from build123d import *

# Parameters (mm, degrees)
SALIENTE_EXTRUIR1_DEPTH = 107
CORTAR_EXTRUIR1_REACH   = 40
CROQUIS3_R              = 2.5
CORTAR_EXTRUIR2_REACH   = 40
CROQUIS4_R              = 2.5


with BuildPart() as part:
    # Croquis1 → Saliente-Extruir1 (new body)
    with BuildSketch(Plane.XY):
        Polygon((0, 0), (9, 0), (17.5, 10.5), (17.5, 24.5), (9, 35), (0, 35), (0, 36.5), (9.715608012, 36.5), (19, 25.031045192), (19, 9.968954808), (9.715608012, -1.5), (0, -1.5), align=None)
    extrude(amount=SALIENTE_EXTRUIR1_DEPTH)

    # Croquis3 → Cortar-Extruir1 (cut, up to next)
    with BuildSketch(Plane(origin=(0, 36.5, 0), x_dir=(1, 0, 0), z_dir=(0, 1, 0)), mode=Mode.PRIVATE) as cortar_extruir1_sk1:
        with Locations((5, -8)):
            Circle(CROQUIS3_R)
    cortar_extruir1_tool1 = extrude(cortar_extruir1_sk1.sketch, amount=-CORTAR_EXTRUIR1_REACH, mode=Mode.PRIVATE) & part.part
    add(cortar_extruir1_tool1.solids().sort_by_distance((5, 36.5, 8))[0], mode=Mode.SUBTRACT)
    # Croquis3 → Cortar-Extruir1 (cut, up to next)
    with BuildSketch(Plane(origin=(0, 36.5, 0), x_dir=(1, 0, 0), z_dir=(0, 1, 0)), mode=Mode.PRIVATE) as cortar_extruir1_sk2:
        with Locations((5, -99)):
            Circle(CROQUIS3_R)
    cortar_extruir1_tool2 = extrude(cortar_extruir1_sk2.sketch, amount=-CORTAR_EXTRUIR1_REACH, mode=Mode.PRIVATE) & part.part
    add(cortar_extruir1_tool2.solids().sort_by_distance((5, 36.5, 99))[0], mode=Mode.SUBTRACT)

    # Croquis4 → Cortar-Extruir2 (cut, up to next)
    with BuildSketch(Plane.XZ.offset(1.5), mode=Mode.PRIVATE) as cortar_extruir2_sk1:
        with Locations((5, 8)):
            Circle(CROQUIS4_R)
    cortar_extruir2_tool1 = extrude(cortar_extruir2_sk1.sketch, amount=-CORTAR_EXTRUIR2_REACH, mode=Mode.PRIVATE) & part.part
    add(cortar_extruir2_tool1.solids().sort_by_distance((5, -1.5, 8))[0], mode=Mode.SUBTRACT)
    # Croquis4 → Cortar-Extruir2 (cut, up to next)
    with BuildSketch(Plane.XZ.offset(1.5), mode=Mode.PRIVATE) as cortar_extruir2_sk2:
        with Locations((5, 99)):
            Circle(CROQUIS4_R)
    cortar_extruir2_tool2 = extrude(cortar_extruir2_sk2.sketch, amount=-CORTAR_EXTRUIR2_REACH, mode=Mode.PRIVATE) & part.part
    add(cortar_extruir2_tool2.solids().sort_by_distance((5, -1.5, 99))[0], mode=Mode.SUBTRACT)


solid = part.part
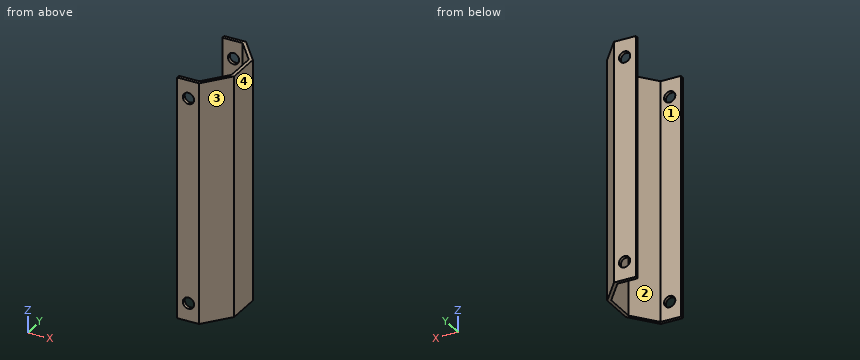
For this review, take the finished solid that the model builds, in its own axes (mm). Face numbers are marked on the shaded views. Round coordinates to 2 decimals unless told otherwise and drop trailing zeros. Loops run counter-clockwise (first coordinate to the right, second up) from the corner with the lowest first, then second, coordinate; pieces in that order, holes last. Notation, with made-up numbers: (21, -13) - (76, -13) arc R11 cw to (76, -3) - close; hole circle Ø2 at (-28.75, 29). An arc over 180 degrees is marked (long way). Put each result on its own line as item: value. Start each with the question number.
1. For probe 1 along Z at (x, y) = (5, 35.6); probe 2 along Y at (x, z) = (3, 96.5); probe 3 along X at (y, z) = (35.95, 8), list the stretches that pass through material, from the lowest coordinate up. Write a range as [from, to].
2. Consider section C-C on z = 58.5. State the section outline as (x, y) points, plus the area to 3 significant figures.
3. Consider section A-A on x = 5. State the section outline as (y, z) points, plus the area to 3 significant figures.
4. Consider section D-D on x = 15. State the section outline as (y, z) points, plus the area to 3 significant figures.
5. Insertion check: P1, Ø1, axis at y = 25, z = 40, coming from the -X side; P2, Ø4, axis at y = 15, z = 76.5, coming from the -X side. Each pin has a flat end and moves straight along its axis. Give the tip position at first contact, or say it passes through.
6. Consider section B-B on z = 99. State the section outline as (x, y) points, plus the area to 3 significant figures.
7. Mouldability with a two-part tool opening along Y and no side actions: class the marked faces 1, 2, 3 and 4 as +Y half, -Y half, draft (parallel to the pull), parting line (faces both ways), or undercut.
Result sheet:
1. probe 1: [0, 5.5], [10.5, 96.5], [101.5, 107]
1. probe 2: [-1.5, 0], [35, 36.5]
1. probe 3: [0, 2.5], [7.5, 10.16]
2. outline: (0, -1.5) - (9.72, -1.5) - (19, 9.97) - (19, 25.03) - (9.72, 36.5) - (0, 36.5) - (0, 35) - (9, 35) - (17.5, 24.5) - (17.5, 10.5) - (9, 0) - (0, 0) - close
2. area: 92.3 mm^2
3. outline: (-1.5, 0) - (0, 0) - (0, 5.5) - (-1.5, 5.5) - close; (-1.5, 10.5) - (0, 10.5) - (0, 96.5) - (-1.5, 96.5) - close; (-1.5, 101.5) - (0, 101.5) - (0, 107) - (-1.5, 107) - close; (35, 0) - (36.5, 0) - (36.5, 5.5) - (35, 5.5) - close; (35, 10.5) - (36.5, 10.5) - (36.5, 96.5) - (35, 96.5) - close; (35, 101.5) - (36.5, 101.5) - (36.5, 107) - (35, 107) - close
3. area: 291 mm^2
4. outline: (5.03, 0) - (7.41, 0) - (7.41, 107) - (5.03, 107) - close; (27.59, 0) - (29.97, 0) - (29.97, 107) - (27.59, 107) - close
4. area: 510 mm^2
5. P1: x = 16.69
5. P2: x = 17.5
6. outline: (0, -1.5) - (2.5, -1.5) - (2.5, 0) - (0, 0) - close; (0, 35) - (2.5, 35) - (2.5, 36.5) - (0, 36.5) - close; (7.5, -1.5) - (9.72, -1.5) - (19, 9.97) - (19, 25.03) - (9.72, 36.5) - (7.5, 36.5) - (7.5, 35) - (9, 35) - (17.5, 24.5) - (17.5, 10.5) - (9, 0) - (7.5, 0) - close
6. area: 77.3 mm^2
7. face 1: undercut
7. face 2: undercut
7. face 3: -Y half
7. face 4: draft
